from build123d import *

# Parameters (mm, degrees)
SKETCH1_W           = 10
SKETCH1_H           = 22
SKETCH1_R           = 4
SKETCH1_R_2         = 2
BOSS_EXTRUDE1_DEPTH = 1.5
CHAMFER1_SIZE       = 0.15


with BuildPart() as part:
    # Sketch1 → Boss-Extrude1 (new, symmetric)
    with BuildSketch(Plane.XY):
        Rectangle(SKETCH1_W, SKETCH1_H)
        Circle(SKETCH1_R, mode=Mode.SUBTRACT)
        with Locations((0, -8)):
            Circle(SKETCH1_R_2, mode=Mode.SUBTRACT)
        with Locations((0, 8)):
            Circle(SKETCH1_R_2, mode=Mode.SUBTRACT)
    extrude(amount=BOSS_EXTRUDE1_DEPTH, both=True)

    # Chamfer1
    chamfer1_edges = [part.edges().sort_by_distance(p)[0] for p in [
        (-4, 0, -1.5),
        (-4, 0, 1.5),
        (5, 0, 1.5),
        (-2, -8, -1.5),
        (-2, -8, 1.5),
        (0, 11, 1.5),
        (-2, 8, -1.5),
        (-2, 8, 1.5),
        (-5, 0, 1.5),
        (0, 11, -1.5),
        (5, 0, -1.5),
        (0, -11, -1.5),
        (-5, 0, -1.5),
        (-5, 11, 0),
        (5, 11, 0),
        (5, -11, 0),
        (-5, -11, 0),
        (0, -11, 1.5),
    ]]
    chamfer(chamfer1_edges, length=CHAMFER1_SIZE)


solid = part.part
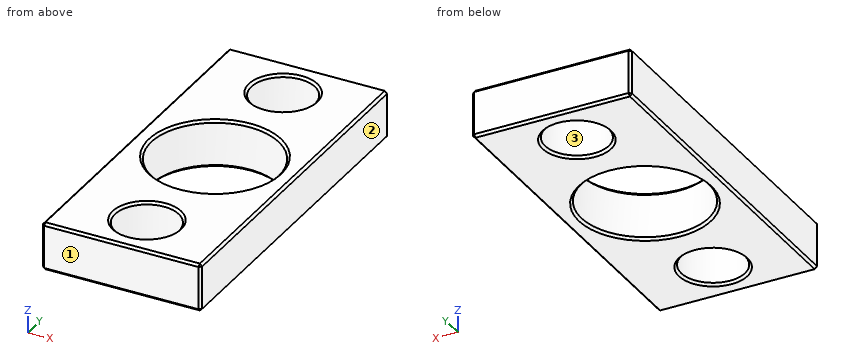
For this review, take the finished solid that the model builds, in its own axes (mm). Face numbers are marked on the shaded views. Round coordinates to 2 decimals unless told otherwise and drop trailing zeros. Loops run counter-clockwise (first coordinate to the right, second up) from the corner with the lowest first, then second, coordinate; pieces in that order, holes last. Notation, with made-up numbers: (-26.5, 26.25) - (-18.5, 26.25) arc R28 cw to (-18.5, 46.25) - close; hole circle Ø11 at (52, -37.75). An arc over 180 degrees is marked (long way). Use one line per item in the form item = value.
1) Mouldability with a two-part tool opening along X and no side actions: class the marked faces 1, 2 and 3 as pulls with the +X half, pulls with the -X half, needs draft (parallel to the pull), parting line crosses it, or undercut.
Solutions:
face_1 = needs draft
face_2 = pulls with the +X half
face_3 = undercut
2) Clearance check with flat-ended pins moving along their axes: P1, Ø4.5, axis at x = 0, y = -8, coming from the +Z side; P2, Ø1, axis at x = 0.5, y = -7, coming from the -Z side. State where each tip first meets the part, or that it passes through.
Solutions:
P1 = 1.5
P2 = through
3) We need section D-D on y = 8. Write out the cut boundary in (x, z), then the cut area to 3 significant figures.
Solutions:
outline = (-5, -1.35) - (-4.85, -1.5) - (-2.15, -1.5) - (-2, -1.35) - (-2, 1.35) - (-2.15, 1.5) - (-4.85, 1.5) - (-5, 1.35) - close; (2, -1.35) - (2.15, -1.5) - (4.85, -1.5) - (5, -1.35) - (5, 1.35) - (4.85, 1.5) - (2.15, 1.5) - (2, 1.35) - close
area = 17.9 mm2
4) Wall thickness on probe 1 along Y at (x, z) = (0, 0.3); probe 2 along Y at (x, z) = (-1, 0.8); probe 3 along X at (y, z) = (2, 0.8): over which ranges is each line inside the solid? List them lowest first.
Solutions:
probe_1 = -11 to -10, -6 to -4, 4 to 6, 10 to 11
probe_2 = -11 to -9.73, -6.27 to -3.87, 3.87 to 6.27, 9.73 to 11
probe_3 = -5 to -3.46, 3.46 to 5
5) We need section C-C on x = 0. State how many separate pieces and enclosed holes the cut face has, then the cut area to 3 significant figures.
Solutions:
separate_pieces = 4
enclosed_holes = 0
area = 17.8 mm2
6) We need section B-B on z = -0.1. Write out the cut boundary in (x, y).
Solutions:
outline = (-5, -10.85) - (-4.85, -11) - (4.85, -11) - (5, -10.85) - (5, 10.85) - (4.85, 11) - (-4.85, 11) - (-5, 10.85) - close; hole circle Ø8 at (0, 0); hole circle Ø4 at (0, -8); hole circle Ø4 at (0, 8)
7) We need section A-A on y = 0. Write out the cut boundary in (x, z), then the cut area to 3 significant figures.
Solutions:
outline = (-5, -1.35) - (-4.85, -1.5) - (-4.15, -1.5) - (-4, -1.35) - (-4, 1.35) - (-4.15, 1.5) - (-4.85, 1.5) - (-5, 1.35) - close; (4, -1.35) - (4.15, -1.5) - (4.85, -1.5) - (5, -1.35) - (5, 1.35) - (4.85, 1.5) - (4.15, 1.5) - (4, 1.35) - close
area = 5.91 mm2
